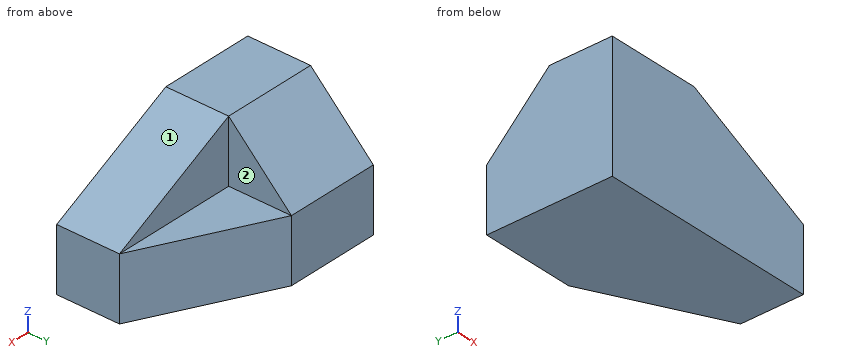
Autodesk Inventor part; units mm, degrees
ref_plane "YZ Plane" through (0, 0, 0) normal (1, 0, 0) x (0, 1, 0)
ref_plane "XZ Plane" through (0, 0, 0) normal (0, 1, 0) x (-1, 0, 0)
ref_plane "XY Plane" through (0, 0, 0) normal (0, 0, 1) x (1, 0, 0)
sketch "草圖1" plane through (0, 0, 0) normal (0, 1, 0) x (-1, 0, 0)
  line L0 (0, 0) -> (-30, 0)
  line L1 (-30, 0) -> (-30, -20)
  line L2 (-30, -20) -> (0, -20)
  line L3 (0, -20) -> (0, 0)
  line L4 (0, -20) -> (-70, -20)
  line L5 (-70, -20) -> (-70, -40)
  line L6 (-70, -40) -> (0, -40)
  line L7 (0, -40) -> (0, -20)
  line L8 (-70, -20) -> (-30, 0)
  dimension "d0" = 70
  dimension "d1" = 20
  dimension "d2" = 20
  dimension "d3" = 30
extrude "擠出1" add sketch "草圖1" along normal blind 20
sketch "草圖2" plane through (0, 0, -40) normal (-1, 0, 0) x (0, 0, 1)
  line L0 (0, 0) -> (0, 20)
  line L1 (0, 20) -> (20, 20)
  line L2 (20, 20) -> (20, 40)
  line L3 (20, 40) -> (0, 40)
  line L4 (0, 40) -> (0, 20)
  line L5 (20, 40) -> (40, 20)
  line L6 (40, 20) -> (20, 20)
  line L7 (40, 20) -> (20, 20)
  point P0 (40, 0)
  dimension "d6" = 20
  dimension "d7" = 20
extrude "擠出2" add sketch "草圖2" against normal blind 30
sketch "草圖3" plane through (70, 0, -40) normal (0, 0, -1) x (-1, 0, 0)
  line L0 (40, 20) -> (40, 40)
  line L1 (0, 20) -> (40, 20)
  line L2 (0, 20) -> (40, 40)
  point P0 (70, 0)
extrude "擠出3" add sketch "草圖3" against normal blind 20
properties part number "13"
The model under review builds one solid part; all positions refer to its coordinate system, in mm. Face numbers are marked on the shaded views. A direction names the side the tool comes from. Round coordinates to 2 decimals unless told otherwise and drop trailing zeros. Order: outer loops, then holes, each group sorted by start corner. A loop starts at its lowest first (then second) coordinate and runs counter-clockwise, first axis right, second up. Notation, with made-up numbers: (20, 1) -> (42, 1) arc R25 cw to (42, 37) -> close; hole circle Ø7 at (-17.5, 60). An arc over 180 degrees is marked (long way). Use CSV: the item, a comma, the result in double quotes. Start each with the question number.
(1) Consider section B-B on z = -31.5. Write out the cut boundary in (x, y), and give its area (3 significant figures).
(2) Tool access review of the marked faces 1 and 2: name each direction out of +Z, -Z, +X, -X, +Y, -Y from which nothing blocks a thin tool from reaching the whole face with its end or side.
(3) Consider section D-D on y = 18. Write out the cut boundary in (x, z).
(4) Consider section A-A on y = 23. Write out the cut boundary in (x, z), and give its area (3 significant figures).
(5) Wall thickness on probe 1 along Z at (x, y) = (49, 21); probe 2 along Y at (x, z) = (37, -4); probe 3 along Z at (x, y) = (13, 23): over which ranges is each line inside the solid? List them lowest first. Write a range as from..to.
(6) Consider section C-C on x = 61. Write out the cut boundary in (y, z).
(7) Insertion check: pin 1 (6 mm diameter, centred on y = 30.5, z = -21.5, fed in from +X); pin 2 (5 mm diameter, centred on y = 24.5, z = -18, fed in from -X); pin 3 (8 mm diameter, centred on x = 35, z = -24.5, fed in from +Y); pin 4 (6 mm diameter, centred on x = 47.5, y = 34.5, fed in from +Z). Each pin has a flat end and moves straight along its axis. Give the tip position at first contact, or say it passes through.
Responses:
1,outline,"(0, 0) -> (70, 0) -> (70, 20) -> (30, 40) -> (0, 40) -> close"
1,area,"2,400 mm²"
2,face 1,"+Z, +X, +Y, -Y"
2,face 2,"+Z, +X, +Y"
3,outline,"(0, -40) -> (70, -40) -> (70, -20) -> (30, 0) -> (0, 0) -> close"
4,outline,"(0, -40) -> (64, -40) -> (64, -20) -> (30, -20) -> (30, -3) -> (0, -3) -> close"
4,area,"1,790 mm²"
5,probe 1,"-40..-20"
5,probe 2,"0..20"
5,probe 3,"-40..-3"
6,outline,"(0, -40) -> (24.5, -40) -> (24.5, -20) -> (20, -20) -> (20, -15.5) -> (0, -15.5) -> close"
7,pin 1,"x = 55"
7,pin 2,"x = 0"
7,pin 3,"y = 39.5"
7,pin 4,"z = -20"
